Could you check a few things on this model? Use its own coordinates, in mm. A direction names the side the tool comes from. Give positions to 0.01 mm unless a question says otherwise; leave off trailing zeros. Write each loop counter-clockwise with the first axis right and the second up, starting at its lowest first coordinate (ties: lowest second). Pieces come first, ordered by that corner, then holes. Notation, with made-up numbers: (-9, 85.25) - (22, 85.25) arc R10 cw to (22, 104.25) - close; hole circle Ø10 at (8.5, 14.25). An arc over 180 degrees is marked (long way). Write item = value, one per line.
from build123d import *

# Parameters (mm, degrees)
BOSS_EXTRUDE2_DEPTH = 10
SKETCH2_R           = 5
CUT_EXTRUDE1_DEPTH  = 192.271419748
SKETCH3_R           = 2.5
SKETCH3_R_2         = 3.112586519
SKETCH3_R_3         = 3.406605284
CUT_EXTRUDE2_DEPTH  = 83.27950738


with BuildPart() as part:
    # Sketch1 → Boss-Extrude2 (new body)
    with BuildSketch(Plane.XY):
        with BuildLine():
            Line((-122.095943171, 24.299679487), (-122.095943171, 54.25))
            Line((-122.095943171, 54.25), (-132.095943171, 54.25))
            Line((-132.095943171, 54.25), (-132.095943171, 34.25))
            Line((-132.095943171, 34.25), (-177.496190175, 12.302884399))
            ThreePointArc((-177.496190175, 12.302884399), (-183.143914757, 3.299679487), (-177.496190175, -5.703525425))
            Line((-177.496190175, -5.703525425), (-132.095943171, -27.650641026))
            Line((-132.095943171, -27.650641026), (-132.095943171, -47.650641026))
            Line((-132.095943171, -47.650641026), (-122.095943171, -47.650641026))
            Line((-122.095943171, -47.650641026), (-122.095943171, -17.700320513))
            ThreePointArc((-122.095943171, -17.700320513), (-143.095943171, 3.299679487), (-122.095943171, 24.299679487))
        make_face()
    extrude(amount=-BOSS_EXTRUDE2_DEPTH)

    # Sketch2 → Cut-Extrude1 (cut, through all)
    with BuildSketch(Plane.XY):
        with Locations((-173.143914757, 3.299679487)):
            Circle(SKETCH2_R)
    extrude(amount=-CUT_EXTRUDE1_DEPTH, mode=Mode.SUBTRACT)

    # Sketch3 → Cut-Extrude2 (cut, through all)
    with BuildSketch(Plane(origin=(-122.095943171, 0, 0), x_dir=(0, 0, -1), z_dir=(1, 0, 0))):
        with Locations((5, 49.25)):
            Circle(SKETCH3_R)
        with Locations((5, 39.25)):
            Circle(SKETCH3_R)
        with Locations((5, -42.650641026)):
            Circle(SKETCH3_R_2)
        with Locations((5, -32.650641026)):
            Circle(SKETCH3_R_3)
    extrude(amount=-CUT_EXTRUDE2_DEPTH, mode=Mode.SUBTRACT)


solid = part.part
1. If we section it at B-B, the plane x = -126.5: Please give me the cut outline in (y, z), and give its area (3 significant figures).
Filled sheet:
outline = (-47.65, -10) - (-17.23, -10) - (-17.23, 0) - (-47.65, 0) - close; (23.83, -10) - (54.25, -10) - (54.25, 0) - (23.83, 0) - close; hole circle Ø6.23 at (-42.65, -5); hole circle Ø6.81 at (-32.65, -5); hole circle Ø5 at (39.25, -5); hole circle Ø5 at (49.25, -5)
area = 502 mm2
2. Thinking about a two-plate mould opening in Y: for faces 1 (the face through (-122.096, -29.6, -2.7)), 2 (the face through (-127, 36.8, -4.5)), 3 (the face through (-127, 54.25, -5)), 4 (the face through (-127.026, -29.273, -4.557)), which applies, pulls with the +Y half, pulls with the -Y half, needs draft (parallel to the pull), parting line crosses it, or undercut?
Filled sheet:
face_1 = needs draft
face_2 = undercut
face_3 = pulls with the +Y half
face_4 = undercut
3. Which directions (+Z, -Z, +X, -X, +Y, -Y) give clear straight access to the entire face, cutting with the end or side of a thin tool? Please do faces 5 (the face through (-132.096, 44, -5)), 6 (the face through (-177.112, 0.257, -4.93)), 7 (the face through (-132.096, -38, -5)).
Filled sheet:
face_5 = +Z, -Z, -X, +Y
face_6 = +Z, -Z
face_7 = +Z, -Z, -X, -Y
4. If we section it at A-A, the plane y = 49.25: Please give me the cut outline in (x, z).
Filled sheet:
outline = (-132.1, -10) - (-122.1, -10) - (-122.1, -7.5) - (-132.1, -7.5) - close; (-132.1, -2.5) - (-122.1, -2.5) - (-122.1, 0) - (-132.1, 0) - close
5. If we section it at D-D, the plane x = -142: Please give me the cut outline in (y, z).
Filled sheet:
outline = (-22.86, -10) - (-3.4, -10) - (-3.4, 0) - (-22.86, 0) - close; (10, -10) - (29.46, -10) - (29.46, 0) - (10, 0) - close
6. For pin 1 (3 mm diameter, centred on y = 42, z = -5.5, fed in from -X); pin 2 (9 mm diameter, centred on x = -173.14, y = 3.3, fed in from +Z); pin 3 (1.5 mm diameter, centred on x = -146.5, z = -8.5, fed in from -Y); pin 4 (1.5 mm diameter, centred on y = 18.5, z = -4.5, fed in from -X), each with a flat end and sliding along its axis, tell me the tip position at first contact or that it passes through.
Filled sheet:
pin_1 = -132.1
pin_2 = through
pin_3 = -21.05
pin_4 = -166.23
7. I need wall thicknesses on line 1 (Y direction, x = -127.5, z = -5); line 2 (Y direction, x = -126, z = -5); line 3 (Y direction, x = -128.5, z = -1.25). Which ranges of each line are inside material? Lowest first, please.
Filled sheet:
line_1 = -47.65 to -45.76, -39.54 to -36.06, -29.24 to -16.99, 23.59 to 36.75, 41.75 to 46.75, 51.75 to 54.25
line_2 = -47.65 to -45.76, -39.54 to -36.06, -29.24 to -17.33, 23.93 to 36.75, 41.75 to 46.75, 51.75 to 54.25
line_3 = -47.65 to -16.7, 23.3 to 54.25
8. If we section it at C-C, the plane z = -5: Please give me the cut outline in (x, y), and give its area (3 significant figures).
Filled sheet:
outline = (-177.5, -5.7) - (-132.1, -27.65) - (-132.1, -29.24) - (-122.1, -29.24) - (-122.1, -17.7) arc R21 cw to (-122.1, 24.3) - (-122.1, 36.75) - (-132.1, 36.75) - (-132.1, 34.25) - (-177.5, 12.3) arc R10 ccw to start; (-132.1, -47.65) - (-122.1, -47.65) - (-122.1, -45.76) - (-132.1, -45.76) - close; (-132.1, -39.54) - (-122.1, -39.54) - (-122.1, -36.06) - (-132.1, -36.06) - close; (-132.1, 41.75) - (-122.1, 41.75) - (-122.1, 46.75) - (-132.1, 46.75) - close; (-132.1, 51.75) - (-122.1, 51.75) - (-122.1, 54.25) - (-132.1, 54.25) - close; hole circle Ø10 at (-173.14, 3.3)
area = 1,900 mm2
